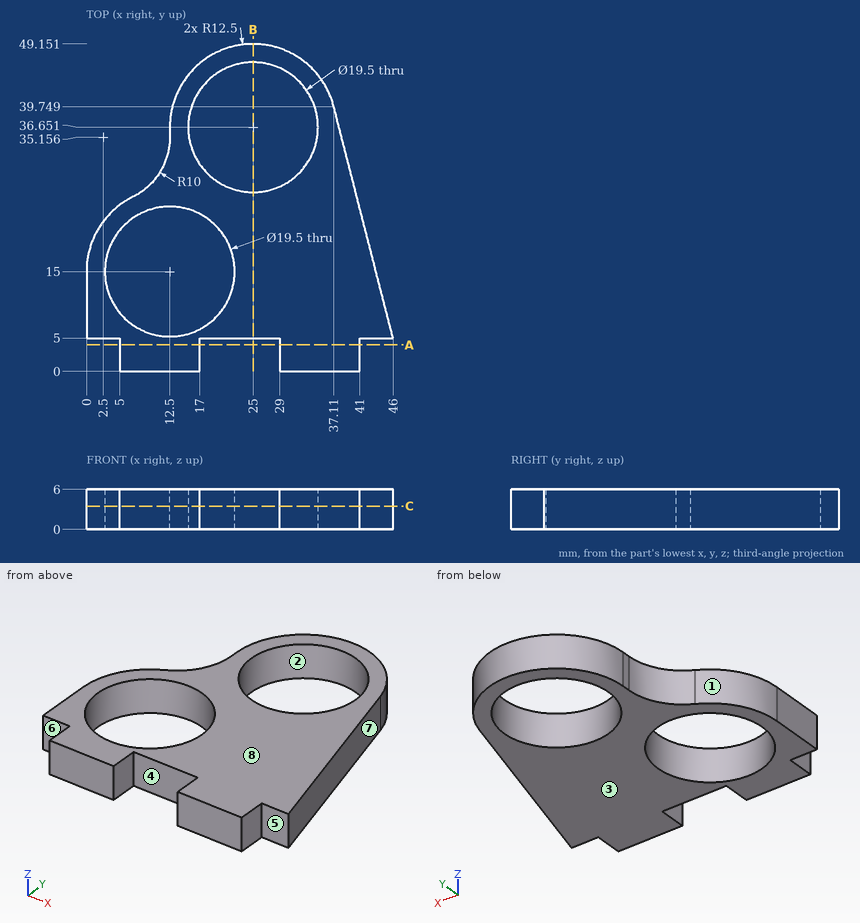
Job drawing, mm, ordinate dimensions from the low corner. One solid piece. A direction names the side the tool comes from. Coordinates: 2 decimals unless noted, no trailing zeros. Loops run counter-clockwise (first coordinate to the right, second up) from the corner with the lowest first, then second, coordinate; pieces in that order, holes last. Notation, with made-up numbers: (48, 68) - (78, 68) arc R18 cw to (78, 82) - close; hole circle Ø4 at (4, -15). An arc over 180 degrees is marked (long way). Answer as a JSON object with one key per item and string values. Group by question number.
(1) Cut at B-B (x = 25). Give the cut face in (y, z), then the cut area to 3 significant figures.
(2) Cut at C-C (z = 3.5). State how many separate pieces and enclosed holes the cut face has.
(3) Tool access for the marked faces 4, 5, 6, 7 and 8: list every direction of +Z, -Z, +X, -X, +Y, -Y with a clear straight run to the whole face (end or side of a thin tool).
(4) Probe line 1 along X through (y, z) = (18, 2.5) (1 decimal); line 2 along Y through (x, z) = (25, 1.55); line 3 along X through (y, z) = (8.5, 2.1) (1 decimal). List the from-to ranges inside material, lowest first.
(5) Cut at A-A (y = 4). Give the cut face in (x, z), then the cut area to 3 significant figures.
(6) Flat gauge pins, fed straight in: pin 1 (15.5 mm diameter, centred on x = 25, y = 36.65, fed in from -Z); pin 2 (2 mm diameter, centred on x = 14, z = 2.5, fed in from +Y); pin 3 (2.5 mm diameter, centred on y = 2.5, z = 1.5, fed in from -X). Where does each tip first touch, or does it go through?
(7) Two-plate mould, pull along X, no slides. Class the marked faces 1, 2 and 3: released by +X, released by -X, zero draft, split by the parting line, or undercut.
Geometry says:
{
 "1": {"outline": "(5, 0) - (26.9, 0) - (26.9, 6) - (5, 6) - close; (46.4, 0) - (49.15, 0) - (49.15, 6) - (46.4, 6) - close", "area": "148 mm^2"},
 "2": {"separate pieces": "1", "enclosed holes": "2"},
 "3": {"face 4": "+Z, -Z, -Y", "face 5": "+Z, -Z, +X, -Y", "face 6": "+Z, -Z, -X, -Y", "face 7": "+Z, -Z, +X, +Y", "face 8": "+Z, +X, -X, +Y, -Y"},
 "4": {"line 1": "x = 0.4 to 3.2, 21.8 to 42.7", "line 2": "y = 5 to 26.9, 46.4 to 49.15", "line 3": "x = 0 to 5.2, 19.8 to 45.1"},
 "5": {"outline": "(5, 0) - (17, 0) - (17, 6) - (5, 6) - close; (29, 0) - (41, 0) - (41, 6) - (29, 6) - close", "area": "144 mm^2"},
 "6": {"pin 1": "passes through", "pin 2": "stops at y = 44.15", "pin 3": "stops at x = 5"},
 "7": {"face 1": "released by -X", "face 2": "undercut", "face 3": "zero draft"}
}
